Verification items for the finished model (mm, model axes). A direction names the side the tool comes from. Round coordinates to 2 decimals unless told otherwise and drop trailing zeros. Write each loop counter-clockwise with the first axis right and the second up, starting at its lowest first coordinate (ties: lowest second). Pieces come first, ordered by that corner, then holes. Notation, with made-up numbers: (47.5, -23.75) -> (74.5, -23.75) arc R22 cw to (74.5, -0.75) -> close; hole circle Ø10 at (69, 54). An arc over 180 degrees is marked (long way). Use CSV: the item, a comma, the result in double quotes.
```python
from build123d import *

# Parameters (mm, degrees)
F0_W     = 45
F0_H     = 26
F1_DEPTH = 26
F2_W     = 24
F2_H     = 24
F3_DEPTH = 45.001
F5_D     = 4.4
F7_D     = 4.4
F9_DEPTH = 2.001
F10_R    = 4


with BuildPart() as f1:
    # F0 (on Top) → F1 (new body)
    with BuildSketch(Plane.XY):
        Rectangle(F0_W, F0_H)
    extrude(amount=F1_DEPTH)

    # F2 (on face) → F3 (cut, through all)
    with BuildSketch(Plane.YZ.offset(22.5)):
        with Locations((-1, 14)):
            Rectangle(F2_W, F2_H)
    extrude(amount=-F3_DEPTH, mode=Mode.SUBTRACT)

    # F5 (through all)
    with Locations(Plane.XY.offset(2)):
        with Locations((-18.5, -9), (18.5, -9)):
            Hole(F5_D / 2)

    # F7 (through all)
    with Locations(Plane.XZ.offset(-11)):
        with Locations((-18.5, 19), (18.5, 19)):
            Hole(F7_D / 2)

    # F8 (on face) → F9 (cut, through all)
    with BuildSketch(Plane.XY.offset(2)):
        with BuildLine():
            ThreePointArc((-12.7, -9), (-10.5, -11.2), (-8.3, -9))
            ThreePointArc((-8.3, -9), (-11.2875108319, -1.7875108319), (-18.5, 1.2))
            ThreePointArc((-18.5, 1.2), (-20.7, -1), (-18.5, -3.2))
            ThreePointArc((-18.5, -3.2), (-14.3987806691, -4.8987806691), (-12.7, -9))
        make_face()
        with BuildLine():
            ThreePointArc((18.5, 1.2), (11.2875108319, -1.7875108319), (8.3, -9))
            ThreePointArc((8.3, -9), (10.5, -11.2), (12.7, -9))
            ThreePointArc((12.7, -9), (14.3987806691, -4.8987806691), (18.5, -3.2))
            ThreePointArc((18.5, -3.2), (20.7, -1), (18.5, 1.2))
        make_face()
    extrude(amount=-F9_DEPTH, mode=Mode.SUBTRACT)

    # F10
    f10_edges = [f1.edges().sort_by_distance(p)[0] for p in [
        (-22.5, -13, 1),
        (22.5, -13, 1),
    ]]
    fillet(f10_edges, radius=F10_R)


solid = f1.part
```
Q1. Section check D-D (x = 18). Record the cut outline in (y, z), plus the area to 3 significant figures.
Filled in:
outline,"(-13, 0) -> (-11.14, 0) -> (-11.14, 2) -> (-13, 2) -> close; (-6.86, 0) -> (-3.22, 0) -> (-3.22, 2) -> (-6.86, 2) -> close; (1.19, 0) -> (13, 0) -> (13, 16.86) -> (11, 16.86) -> (11, 2) -> (1.19, 2) -> close; (11, 21.14) -> (13, 21.14) -> (13, 26) -> (11, 26) -> close"
area,"74.0 mm²"
Q2. Go/stop test with flat-tipped pins: P1, Ø12, axis at x = -2, z = 11.5, coming from the -Y side; P2, Ø7, axis at x = 10, y = -1, coming from the +Z side. Record where each tip stops, or that it passes through.
Filled in:
P1,"y = 11"
P2,"z = 2"
Q3. Mould release check, pull along X, two halves, no side actions. Record for faces 4 (the cylindrical face through (-14.4, -4.9, 1)), 5 (the flat face through (-22.5, 12, 7)), 6 (the flat face through (0, 12, 26)), 7 (the cylindrical face through (21.297, -11.859, 1.014)): released by +X, released by -X, zero draft, split by the parting line, or undercut.
Filled in:
face 4,"undercut"
face 5,"released by -X"
face 6,"zero draft"
face 7,"released by +X"
Q4. Section check A-A (z = 19). Record the cut outline in (x, y).
Filled in:
outline,"(-22.5, 11) -> (-20.7, 11) -> (-20.7, 13) -> (-22.5, 13) -> close; (-16.3, 11) -> (16.3, 11) -> (16.3, 13) -> (-16.3, 13) -> close; (20.7, 11) -> (22.5, 11) -> (22.5, 13) -> (20.7, 13) -> close"
Q5. Material ranges on L1, parallel to Y at x = -18.5, z = 0.5; L2, parallel to Z at x = -18.5, y = 11.6; L3, parallel to Y at x = 5, z = 13.75, recorded low to high.
Filled in:
L1,"-13 to -11.2, -6.8 to -3.2, 1.2 to 13"
L2,"0 to 16.8, 21.2 to 26"
L3,"11 to 13"
Q6. Section check B-B (x = 10.5). Record the cut outline in (y, z), plus the area to 3 significant figures.
Filled in:
outline,"(-13, 0) -> (-11.2, 0) -> (-11.2, 2) -> (-13, 2) -> close; (-2.67, 0) -> (13, 0) -> (13, 26) -> (11, 26) -> (11, 2) -> (-2.67, 2) -> close"
area,"82.9 mm²"
Q7. Section check C-C (y = -1). Record the cut outline in (x, z), plus the area to 3 significant figures.
Filled in:
outline,"(-22.5, 0) -> (-20.7, 0) -> (-20.7, 2) -> (-22.5, 2) -> close; (-12.17, 0) -> (12.17, 0) -> (12.17, 2) -> (-12.17, 2) -> close; (20.7, 0) -> (22.5, 0) -> (22.5, 2) -> (20.7, 2) -> close"
area,"55.9 mm²"
Q8. Access from +Z, -Z, +X, -X, +Y, -Y to the whole of each face (thin tool, end or side, straight path). Record for faces 1 (the cylindrical face through (-20.532, 12.014, 18.157)), 2 (the cylindrical face through (-10.5, -11.2, 1)), 3 (the flat face through (0, -1, 2)).
Filled in:
face 1,"+Y, -Y"
face 2,"+Z, -Z"
face 3,"+Z, +X, -X, -Y"
